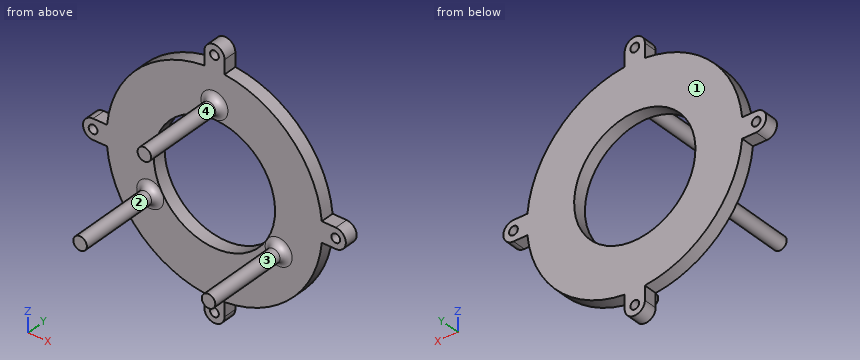
from build123d import *

# Parameters (mm, degrees)
SKETCH1_R           = 1
BOSS_EXTRUDE1_DEPTH = 13
SKETCH2_R           = 9
SKETCH2_R_2         = 0.65
BOSS_EXTRUDE2_DEPTH = 2
CIRPATTERN2_COUNT   = 3
FILLET1_R           = 1


with BuildPart() as part:
    # Sketch1 → Boss-Extrude1 (new body)
    with BuildSketch(Plane(origin=(0, 0, 0), x_dir=(1, 0, 0), z_dir=(0, 1, 0))):
        with Locations(Location((0, -11, 0), (0, 0, 270))):
            Circle(SKETCH1_R)
    boss_extrude1 = extrude(amount=-BOSS_EXTRUDE1_DEPTH)

    # Sketch2 → Boss-Extrude2 (add)
    with BuildSketch(Plane(origin=(0, 0, 0), x_dir=(1, 0, 0), z_dir=(0, 1, 0))):
        with BuildLine():
            Line((-18, 1.5), (-15.929532322, 1.5))
            ThreePointArc((-15.929532322, 1.5), (-11.313708499, 11.313708499), (-1.5, 15.929532322))
            Line((-1.5, 15.929532322), (-1.5, 18))
            ThreePointArc((-1.5, 18), (0, 19.5), (1.5, 18))
            Line((1.5, 18), (1.5, 15.929532322))
            ThreePointArc((1.5, 15.929532322), (11.313708499, 11.313708499), (15.929532322, 1.5))
            Line((15.929532322, 1.5), (18, 1.5))
            ThreePointArc((18, 1.5), (19.5, 0), (18, -1.5))
            Line((18, -1.5), (15.929532322, -1.5))
            ThreePointArc((15.929532322, -1.5), (11.313708499, -11.313708499), (1.5, -15.929532322))
            Line((1.5, -15.929532322), (1.5, -18))
            ThreePointArc((1.5, -18), (0, -19.5), (-1.5, -18))
            Line((-1.5, -18), (-1.5, -15.929532322))
            ThreePointArc((-1.5, -15.929532322), (-11.313708499, -11.313708499), (-15.929532322, -1.5))
            Line((-15.929532322, -1.5), (-18, -1.5))
            ThreePointArc((-18, -1.5), (-19.5, 0), (-18, 1.5))
        make_face()
        with Locations(Location((0, 0, 0), (0, 0, 270))):
            Circle(SKETCH2_R, mode=Mode.SUBTRACT)
        with Locations(Location((0, 18, 0), (0, 0, 270))):
            Circle(SKETCH2_R_2, mode=Mode.SUBTRACT)
        with Locations(Location((18, 0, 0), (0, 0, 270))):
            Circle(SKETCH2_R_2, mode=Mode.SUBTRACT)
        with Locations(Location((-18, 0, 0), (0, 0, 270))):
            Circle(SKETCH2_R_2, mode=Mode.SUBTRACT)
        with Locations(Location((0, -18, 0), (0, 0, 270))):
            Circle(SKETCH2_R_2, mode=Mode.SUBTRACT)
    extrude(amount=BOSS_EXTRUDE2_DEPTH)

    # CirPattern2: Boss-Extrude1 ×3 about axis
    cirpattern2_axis = Axis((0, 0, 0), (0, 1, 0))
    for i in range(1, CIRPATTERN2_COUNT):
        add(boss_extrude1.rotate(cirpattern2_axis, i * 360 / CIRPATTERN2_COUNT))

    # Fillet1
    fillet1_edges = [part.edges().sort_by_distance(p)[0] for p in [
        (0, 0, 10),
        (8.660254038, 0, -5),
        (-8.660254038, 0, -5),
    ]]
    fillet(fillet1_edges, radius=FILLET1_R - 0.0001)  # a hair under: the kernel refuses the full size


solid = part.part
Build history of the part. All positions in model axes, mm. Face numbers are marked on the shaded views. Give positions to 0.01 mm unless a question says otherwise; leave off trailing zeros. Order: outer loops, then holes, each group sorted by start corner. A loop starts at its lowest first (then second) coordinate and runs counter-clockwise, first axis right, second up. Notation, with made-up numbers: M 16.25,79.25 L 24.25,79.25 A16 cw 24.25,86.25 Z; hole C 39.5,-2 d8. An arc over 180 degrees is marked long. Put each result on its own line as item: value.
Item 1: Cut at C-C on y = 0.5. Write the cut outline in (x, z), then the cut area to 3 significant figures.
Results are:
outline: M -18,-1.5 L -15.93,-1.5 A16 ccw -1.5,-15.93 L -1.5,-18 A1.5 ccw 1.5,-18 L 1.5,-15.93 A16 ccw 15.93,-1.5 L 18,-1.5 A1.5 ccw 18,1.5 L 15.93,1.5 A16 ccw 1.5,15.93 L 1.5,18 A1.5 ccw -1.5,18 L -1.5,15.93 A16 ccw -15.93,1.5 L -18,1.5 A1.5 ccw Z; hole C -18,0 d1.3; hole C 0,0 d18; hole C 0,-18 d1.3; hole C 0,18 d1.3; hole C 18,0 d1.3
area: 583 mm2
Item 2: Drop flat-ended pins along their axis: pin 1 Ø1 at (x, y) = (17.5, 1) entering from +Z; pin 2 Ø8 at (x, y) = (-15.5, -10.5) entering from +Z; pin 3 Ø0.6 at (x, y) = (17, 1) entering from -Z; pin 4 Ø2 at (x, z) = (-18, 0) entering from -Y. Give the stop position or say it passes through.
Results are:
pin 1: z = 1.5
pin 2: through
pin 3: z = -1.5
pin 4: y = 0
Item 3: Cut at B-B on z = 0. Write the cut outline in (x, y), then the cut area to 3 significant figures.
Results are:
outline: M -19.5,0 L -18.65,0 L -18.65,2 L -19.5,2 Z; M -17.35,0 L -9,0 L -9,2 L -17.35,2 Z; M 9,0 L 17.35,0 L 17.35,2 L 9,2 Z; M 18.65,0 L 19.5,0 L 19.5,2 L 18.65,2 Z
area: 36.8 mm2
Item 4: Pull direction X, two halves, no side cores. Call the marked faces 1, 2, 3 and 4: +X half, -X half, draft (parallel to the pull), parting line (faces both ways), or undercut.
Results are:
face 1: draft
face 2: undercut
face 3: undercut
face 4: parting line
Item 5: Cut at D-D on z = 4. Write the cut outline in (x, y), then the cut area to 3 significant figures.
Results are:
outline: M -15.49,0 L -8.06,0 L -8.06,2 L -15.49,2 Z; M 8.06,0 L 15.49,0 L 15.49,2 L 8.06,2 Z
area: 29.7 mm2
Item 6: Cut at A-A on x = 0. Count the separate pieces of the cut face and the enclosed holes in it, then the cut area to 3 significant figures.
Results are:
separate pieces: 4
enclosed holes: 0
area: 63.2 mm2
Item 7: Wall check: probe 1 along X at (y, z) = (1.15, 0); probe 2 along X at (y, z) = (1.6, 18); probe 3 along Y at (x, z) = (15.5, 0). Give the ranges that are in metal, low to high.
Results are:
probe 1: -19.5 to -18.65, -17.35 to -9, 9 to 17.35, 18.65 to 19.5
probe 2: -1.5 to -0.65, 0.65 to 1.5
probe 3: 0 to 2
